```python
from build123d import *

# Parameters (mm, degrees)
SKETCH1_R           = 31
SKETCH1_R_2         = 2
BOSS_EXTRUDE1_DEPTH = 1
FILLET1_R           = 10


with BuildPart() as part:
    # Sketch1 → Boss-Extrude1 (new, symmetric)
    with BuildSketch(Plane.XY):
        with BuildLine():
            Line((-41.821047333, 10), (-98.5, 10))
            Line((-98.5, 10), (-98.5, -10))
            Line((-98.5, -10), (-41.821047333, -10))
            ThreePointArc((-41.821047333, -10), (0, -43), (41.821047333, -10))
            Line((41.821047333, -10), (98.5, -10))
            Line((98.5, -10), (98.5, 10))
            Line((98.5, 10), (41.821047333, 10))
            ThreePointArc((41.821047333, 10), (0, 43), (-41.821047333, 10))
        make_face()
        Circle(SKETCH1_R, mode=Mode.SUBTRACT)
        with Locations((0, 38.5)):
            Circle(SKETCH1_R_2, mode=Mode.SUBTRACT)
        with Locations((27.223611076, 27.223611076)):
            Circle(SKETCH1_R_2, mode=Mode.SUBTRACT)
        with Locations((38.5, 0)):
            Circle(SKETCH1_R_2, mode=Mode.SUBTRACT)
        with Locations((27.223611076, -27.223611076)):
            Circle(SKETCH1_R_2, mode=Mode.SUBTRACT)
        with Locations((0, -38.5)):
            Circle(SKETCH1_R_2, mode=Mode.SUBTRACT)
        with Locations((-27.223611076, -27.223611076)):
            Circle(SKETCH1_R_2, mode=Mode.SUBTRACT)
        with Locations((-38.5, 0)):
            Circle(SKETCH1_R_2, mode=Mode.SUBTRACT)
        with Locations((-27.223611076, 27.223611076)):
            Circle(SKETCH1_R_2, mode=Mode.SUBTRACT)
        with Locations((-58.5, 0)):
            Circle(SKETCH1_R_2, mode=Mode.SUBTRACT)
        with Locations((-88.5, 0)):
            Circle(SKETCH1_R_2, mode=Mode.SUBTRACT)
        with Locations((58.5, 0)):
            Circle(SKETCH1_R_2, mode=Mode.SUBTRACT)
        with Locations((88.5, 0)):
            Circle(SKETCH1_R_2, mode=Mode.SUBTRACT)
    extrude(amount=BOSS_EXTRUDE1_DEPTH, both=True)

    # Fillet1
    fillet1_edges = [part.edges().sort_by_distance(p)[0] for p in [
        (98.5, -10, 0),
        (98.5, 10, 0),
        (41.821047333, -10, 0),
        (41.821047333, 10, 0),
        (-41.821047333, -10, 0),
        (-98.5, -10, 0),
        (-98.5, 10, 0),
        (-41.821047333, 10, 0),
    ]]
    fillet(fillet1_edges, radius=FILLET1_R - 0.0001)  # a hair under: the kernel refuses the full size


solid = part.part
```
Can you work these out from the model? Positions are in its coordinate system, mm. Give positions to 0.01 mm unless a question says otherwise; leave off trailing zeros. Write each loop counter-clockwise with the first axis right and the second up, starting at its lowest first coordinate (ties: lowest second). Pieces come first, ordered by that corner, then holes. Notation, with made-up numbers: (-36, 58.5) -> (1, 58.5) arc R36 ccw to (1, 95.5) -> close; hole circle Ø5 at (-40, 56.5). An arc over 180 degrees is marked (long way). One line per item, written item: value.
Q1. For P1, Ø1, axis at x = -14, z = 0, coming from the +Y side; P2, Ø0.6, axis at x = -76.5, z = -0.5, coming from the -Y side; P3, Ø1, axis at x = -60.5, z = -0.5, coming from the +Y side, each with a flat end and sliding along its axis, tell me the tip position at first contact or that it passes through.
Results found:
P1: stops at y = 40.83
P2: stops at y = -10
P3: stops at y = 10
Q2. Imagine slicing it at B-B on y = -19. Please give me the cut outline in (x, z).
Results found:
outline: (-38.57, -1) -> (-24.49, -1) -> (-24.49, 1) -> (-38.57, 1) -> close; (24.49, -1) -> (38.57, -1) -> (38.57, 1) -> (24.49, 1) -> close
Q3. Imagine slicing it at A-A on x = -58.5. Please give me the cut outline in (y, z), and give its area (3 significant figures).
Results found:
outline: (-10, -1) -> (-2, -1) -> (-2, 1) -> (-10, 1) -> close; (2, -1) -> (10, -1) -> (10, 1) -> (2, 1) -> close
area: 32.0 mm^2
Q4. Please list where these lines run through material, in increasing order: line 1 (Y direction, x = 0, z = -0.45); line 2 (Y direction, x = -58.5, z = 0.1); line 3 (Y direction, x = 50, z = 0.1). Write a range as [from, to].
Results found:
line 1: y = [-43, -40.5], [-36.5, -31], [31, 36.5], [40.5, 43]
line 2: y = [-10, -2], [2, 10]
line 3: y = [-10, 10]
Q5. We'd pull the mould along Y, two halves only. Please class faces 1 (the face through (95.49, 7.15, -0.01)), 2 (the face through (-30, 10, 1)), 3 (the face through (36.502, 0.088, -0.014)): +Y half, -Y half, draft (parallel to the pull), parting line (faces both ways), or undercut.
Results found:
face 1: +Y half
face 2: draft
face 3: undercut
Q6. Imagine slicing it at C-C on x = 0. Please give me the cut outline in (y, z).
Results found:
outline: (-43, -1) -> (-40.5, -1) -> (-40.5, 1) -> (-43, 1) -> close; (-36.5, -1) -> (-31, -1) -> (-31, 1) -> (-36.5, 1) -> close; (31, -1) -> (36.5, -1) -> (36.5, 1) -> (31, 1) -> close; (40.5, -1) -> (43, -1) -> (43, 1) -> (40.5, 1) -> close
Q7. Imagine slicing it at D-D on z = -0.4. Give the number of separate pieces and of enclosed holes in the cut face, and give its area (3 significant figures).
Results found:
separate pieces: 1
enclosed holes: 13
area: 4,830 mm^2
